```python
from build123d import *

# Parameters (mm, degrees)
PAD_DEPTH    = 3
PAD001_DEPTH = 3
SKETCH002_W  = 209.08447
SKETCH002_H  = 4.18
PAD002_DEPTH = 3


with BuildPart() as part:
    # Sketch → Pad (new body)
    with BuildSketch(Plane.XY):
        with BuildLine():
            ThreePointArc((-100, 45), (-145, 0), (-100, -45))
            Line((-100, -45), (100, -45))
            ThreePointArc((100, -45), (145, 0), (100, 45))
            Line((-100, 45), (100, 45))
        make_face()
    extrude(amount=PAD_DEPTH)

    # Sketch001 (on Face6 of Pad) → Pad001 (join)
    with BuildSketch(Plane.XY.offset(3)):
        with BuildLine():
            ThreePointArc((-100, 45), (-145, 0), (-100, -45))
            Line((-100, -45), (100, -45))
            ThreePointArc((100, -45), (145, 0), (100, 45))
            Line((-100, 45), (100, 45))
        make_face()
        with BuildLine():
            ThreePointArc((-100, 5), (-105, 0), (-100, -5))
            Line((-100, -5), (100, -5))
            ThreePointArc((100, -5), (105, 0), (100, 5))
            Line((-100, 5), (100, 5))
        make_face(mode=Mode.SUBTRACT)
    extrude(amount=PAD001_DEPTH)

    # Sketch002 (on Face9 of Pad001) → Pad002 (join)
    with BuildSketch(Plane.XY.offset(6)):
        with BuildLine():
            ThreePointArc((-100, 45), (-145, 0), (-100, -45))
            Line((-100, -45), (100, -45))
            ThreePointArc((100, -45), (145, 0), (100, 45))
            Line((-100, 45), (100, 45))
        make_face()
        Rectangle(SKETCH002_W, SKETCH002_H, mode=Mode.SUBTRACT)
    extrude(amount=PAD002_DEPTH)


solid = part.part
```
Can you work these out from the model? Positions are in its coordinate system, mm. A direction names the side the tool comes from. Round coordinates to 2 decimals unless told otherwise and drop trailing zeros. Order: outer loops, then holes, each group sorted by start corner. A loop starts at its lowest first (then second) coordinate and runs counter-clockwise, first axis right, second up.
(1) I'm going to push flat-ended pins straight in: pin 1 (2.5 mm diameter, centred on x = -4, y = 4, fed in from -Z); pin 2 (2.5 mm diameter, centred on y = 0, z = 7.5, fed in from +X); pin 3 (2.5 mm diameter, centred on y = -0.5, z = 7, fed in from -X). Where does each tip first touch, or does it pass through?
Results are:
pin 1: stops at z = 0
pin 2: stops at x = 145
pin 3: stops at x = -145
(2) If we section it at B-B (y = -35.5): Please give me the cut outline in (x, z).
Results are:
outline: (-127.65, 0) - (127.65, 0) - (127.65, 9) - (-127.65, 9) - close
(3) On a 3-axis mill with a long thin cutter (end or side, diameter ignored), from which of +Z, -Z, +X, -X, +Y, -Y can I reach the whole of each face in a straight line? I mean faces 4 (the face through (-1, -45, 4)), 5 (the face through (105, 0, 4)). Say none if no direction works.
Results are:
face 4: +Z, -Z, +X, -X, -Y
face 5: none
(4) If I drill on L1, parallel to Y at x = -96.5, z = 5.5; L2, parallel to Z at x = 55, y = -3.5; L3, parallel to Y at x = 102.5, z = 8, over which ranges is the centre line in solid material (lowest first)?
Results are:
L1: y = -45 to -5, 5 to 45
L2: z = 0 to 3, 6 to 9
L3: y = -44.93 to -2.09, 2.09 to 44.93
(5) If we section it at A-A (x = -52): Please give me the cut outline in (y, z), plus the area to 3 significant figures.
Results are:
outline: (-45, 0) - (45, 0) - (45, 9) - (2.09, 9) - (2.09, 6) - (5, 6) - (5, 3) - (-5, 3) - (-5, 6) - (-2.09, 6) - (-2.09, 9) - (-45, 9) - close
area: 767 mm2
(6) If we section it at C-C (y = 15): Please give me the cut outline in (x, z), plus the area to 3 significant figures.
Results are:
outline: (-142.43, 0) - (142.43, 0) - (142.43, 9) - (-142.43, 9) - close
area: 2,560 mm2
(7) We'd pull the mould along Y, two halves only. Please class faces 1 (the face through (-105, 0, 4)), 2 (the face through (-2, 1, 0)), 3 (the face through (-144.99, 0.99, 4.44)): +Y half, -Y half, draft (parallel to the pull), parting line (faces both ways), or undercut.
Results are:
face 1: undercut
face 2: draft
face 3: parting line
